from build123d import *

# Parameters (mm, degrees)
SKETCH1_W           = 40
SKETCH1_H           = 30
BOSS_EXTRUDE1_DEPTH = 7
SKETCH2_W           = 36
SKETCH2_H           = 26
CUT_EXTRUDE1_DEPTH  = 5
FILLET1_R           = 2
FILLET2_R           = 2
SKETCH3_W           = 7
SKETCH3_H           = 4
CUT_EXTRUDE2_DEPTH  = 2
CUT_EXTRUDE3_REACH  = 51.325
SKETCH6_W           = 10.5
SKETCH6_H           = 4.355980474
SKETCH7_W           = 2
SKETCH7_H           = 2
CUT_EXTRUDE4_DEPTH  = 10


with BuildPart() as part:
    # Sketch1 → Boss-Extrude1 (new body)
    with BuildSketch(Plane.XY):
        with Locations((20, 15)):
            Rectangle(SKETCH1_W, SKETCH1_H)
    extrude(amount=BOSS_EXTRUDE1_DEPTH)

    # Sketch2 → Cut-Extrude1 (cut)
    with BuildSketch(Plane.XY.offset(7)):
        with Locations((20, 15)):
            Rectangle(SKETCH2_W, SKETCH2_H)
    extrude(amount=-CUT_EXTRUDE1_DEPTH, mode=Mode.SUBTRACT)

    # Fillet1
    fillet1_edges = [part.edges().sort_by_distance(p)[0] for p in [
        (2, 2, 4.5),
        (2, 28, 4.5),
    ]]
    fillet(fillet1_edges, radius=FILLET1_R)

    # Fillet2
    fillet2_edges = [part.edges().sort_by_distance(p)[0] for p in [
        (40, 15, 7),
        (20, 30, 7),
        (0, 15, 7),
        (20, 0, 7),
        (0, 30, 3.5),
        (40, 30, 3.5),
        (40, 0, 3.5),
        (0, 0, 3.5),
    ]]
    fillet(fillet2_edges, radius=FILLET2_R - 0.0001)  # a hair under: the kernel refuses the full size

    # Sketch3 → Cut-Extrude2 (cut)
    with BuildSketch(Plane.XY.offset(2)):
        with Locations((34.5, 4)):
            Rectangle(SKETCH3_W, SKETCH3_H)
    extrude(amount=-CUT_EXTRUDE2_DEPTH, mode=Mode.SUBTRACT)

    # Cut-Extrude3: up to this face of the body (flat: up to its plane)
    cut_extrude3_end = Plane(part.part.faces().sort_by_distance((20, 0, 2.50005))[0])
    # Sketch6 → Cut-Extrude3 (cut, up to the picked face)
    with BuildSketch(Plane(origin=(0, 2, 0), x_dir=(1, 0, 0), z_dir=(0, 1, 0)), mode=Mode.PRIVATE) as cut_extrude3_sk1:
        with Locations((20.475771031, -4.177990237)):
            Rectangle(SKETCH6_W, SKETCH6_H)
    cut_extrude3_tool1 = split(extrude(cut_extrude3_sk1.sketch, amount=-CUT_EXTRUDE3_REACH, mode=Mode.PRIVATE), bisect_by=cut_extrude3_end, keep=Keep.BOTH, mode=Mode.PRIVATE)
    add(cut_extrude3_tool1.solids().sort_by(Axis((20.475771, 2, 4.17799), (0, -1, 0)))[0], mode=Mode.SUBTRACT)

    # Sketch7 → Cut-Extrude4 (cut)
    with BuildSketch(Plane(origin=(0, 0, 0), x_dir=(-1, 0, 0), z_dir=(0, 0, -1))):
        with Locations((-39, 4)):
            Rectangle(SKETCH7_W, SKETCH7_H)
    extrude(amount=-CUT_EXTRUDE4_DEPTH, mode=Mode.SUBTRACT)


solid = part.part
Can you work these out from the model? Positions are in its coordinate system, mm. A direction names the side the tool comes from. Give positions to 0.01 mm unless a question says otherwise; leave off trailing zeros. Loops run counter-clockwise (first coordinate to the right, second up) from the corner with the lowest first, then second, coordinate; pieces in that order, holes last. Notation, with made-up numbers: (51, -17) - (83, -17) arc R10 cw to (83, -1) - close; hole circle Ø3 at (-26, 19). An arc over 180 degrees is marked (long way). Answer as a JSON object with one key per item and string values.
Q1. Imagine slicing it at C-C on z = 5.75. Write out the boundary of the cut face in (x, y), plus the area to 3 significant figures.
Geometry says:
{"outline": "(0.15, 2) arc R1.85 ccw to (2, 0.15) - (15.23, 0.15) - (15.23, 2) - (4, 2) arc R2 cw to (2, 4) - (2, 26) arc R2 cw to (4, 28) - (38, 28) - (38, 5) - (39.85, 5) - (39.85, 28) arc R1.85 ccw to (38, 29.85) - (2, 29.85) arc R1.85 ccw to (0.15, 28) - close; (25.73, 0.15) - (38, 0.15) arc R1.85 ccw to (39.85, 2) - (39.85, 3) - (38, 3) - (38, 2) - (25.73, 2) - close", "area": "219 mm²"}
Q2. If I drill on L1, parallel to X at y = 13.25, z = 3.75; L2, parallel to Y at x = 6, z = 3.25; L3, parallel to Y at x = 37, z = 1, over which ranges is the centre line in solid material (lowest first)?
Geometry says:
{"L1": "0 to 2, 38 to 40", "L2": "0 to 2, 28 to 30", "L3": "0 to 2, 6 to 30"}
Q3. If we mould it in two halves opening along Y, with no side actions, what happens to faces 5 (the cylindrical face through (20.25, 29.4, 6.43)), 6 (the flat face through (0, 15, 2)), 7 (the cylindrical face through (20.25, 0.87, 6.65)), 8 (the flat face through (31, 4, 1))? For each: pulls with the +Y half, pulls with the -Y half, needs draft (parallel to the pull), parting line crosses it, or undercut.
Geometry says:
{"face 5": "pulls with the +Y half", "face 6": "needs draft", "face 7": "pulls with the -Y half", "face 8": "undercut"}
Q4. Which directions (+Z, -Z, +X, -X, +Y, -Y) give clear straight access to the entire face, cutting with the end or side of a thin tool? Please do faces 1 (the flat face through (15.226, 1, 4)), 2 (the flat face through (34, 6, 1)), 3 (the flat face through (39, 3, 3)), 4 (the flat face through (21, 28, 5)).
Geometry says:
{"face 1": "-Y", "face 2": "+Z, -Z", "face 3": "+Z, -Z, +X", "face 4": "+Z"}
Q5. Will these pins go through, and if not, where does the flat tip stop? P1, Ø1.6, axis at x = 39, z = 3, coming from the +Y side; P2, Ø0.6, axis at y = 0.5, z = 5, coming from the +X side; P3, Ø1.5, axis at x = 35, y = 21, coming from the +Z side.
Geometry says:
{"P1": "y = 29.99", "P2": "x = 39.6", "P3": "z = 2"}
